```python
from build123d import *

# Parameters (mm, degrees)
SKETCH_1_R               = 13
SKETCH_1_R_2             = 12
EXTRUDE_1_DEPTH          = 6
SKETCH_2_R               = 0.75
CUT_EXTRUDE_1_DEPTH      = 14
PATTERN_CIRCULAR_1_COUNT = 16
SKETCH_3_W               = 36.79853237
SKETCH_3_H               = 11.94610836
CUT_EXTRUDE_2_DEPTH      = 14.0000001


with BuildPart() as part:
    # ｽｹｯﾁ1 → ﾎﾞｽ - 押し出し1 (new body)
    with BuildSketch(Plane.XY):
        Circle(SKETCH_1_R)
        Circle(SKETCH_1_R_2, mode=Mode.SUBTRACT)
    extrude(amount=EXTRUDE_1_DEPTH)

    # ｽｹｯﾁ2 → ｶｯﾄ - 押し出し1 (cut, through all)
    with BuildSketch(Plane(origin=(0, 0, 0), x_dir=(1, 0, 0), z_dir=(0, 1, 0))):
        with Locations((0, -3)):
            Circle(SKETCH_2_R)
    cut_extrude_1 = extrude(amount=-CUT_EXTRUDE_1_DEPTH, mode=Mode.SUBTRACT)

    # 円形ﾊﾟﾀｰﾝ1: ｶｯﾄ - 押し出し1 ×16 about axis
    pattern_circular_1_axis = Axis((0, 0, 0), (0, 0, 1))
    for i in range(1, PATTERN_CIRCULAR_1_COUNT):
        add(cut_extrude_1.rotate(pattern_circular_1_axis, i * 360 / PATTERN_CIRCULAR_1_COUNT), mode=Mode.SUBTRACT)

    # ｽｹｯﾁ3 → ｶｯﾄ - 押し出し2 (cut, through all)
    with BuildSketch(Plane(origin=(0, 0, 0), x_dir=(1, 0, 0), z_dir=(0, 1, 0))):
        with Locations((0, -2.028241391)):
            Rectangle(SKETCH_3_W, SKETCH_3_H)
    extrude(amount=-CUT_EXTRUDE_2_DEPTH, mode=Mode.SUBTRACT)


solid = part.part
```
Source: CAD feature listing. Evaluate the final solid. Frame: model axes, mm. Coordinates: 2 decimals unless noted, no trailing zeros. Loops run counter-clockwise (first coordinate to the right, second up) from the corner with the lowest first, then second, coordinate; pieces in that order, holes last. Notation, with made-up numbers: M 89,-24 L 127,-24 A13 ccw 127,-15 Z; hole C 58,-0.5 d10. An arc over 180 degrees is marked long. Put each result on its own line as item: value. Start each with the question number.
1) Ray query, L1, parallel to Z at x = 0, y = 12.6; L2, parallel to X at y = 4.75, z = 4.25; L3, parallel to X at y = 1.75, z = 1. Return the intervals inside material, ascending. Write a range as from..to.
2) Cut plane B-B on z = 3. Give the number of separate pieces and of enclosed holes in the cut face, then the cut area to 3 significant figures.
3) Contact query for flat-ended pins moving along their axis: pin 1 Ø4 at (x, y) = (9, 3.5) entering from +Z; pin 2 Ø1 at (x, z) = (7, 3.5) entering from -Y; pin 3 Ø3 at (x, y) = (-0.5, 11.5) entering from -Z; pin 4 Ø1.5 at (x, z) = (-5.5, 3) entering from -Y. Output: stop coordinate, or through.
4) Pull-direction query (Y, two-part tool) for faces 1 (the face through (0, 12, 2)), 2 (the face through (-9.33, 8.32, 2.77)), 3 (the face through (0.163, 12.481, 3.732)); classes: pulls with the +Y half, pulls with the -Y half, needs draft (parallel to the pull), parting line crosses it, or undercut.
5) Cut plane A-A on x = 0. Return the cut outline in (y, z), then the cut area to 3 significant figures.
6) Cut plane C-C on y = 1.25. Return the cut outline in (x, z), then the cut area to 3 significant figures.
7) Cut plane D-D on z = 5.5. Return the cut outline in (x, y), then the cut area to 3 significant figures.
The answers:
1. L1: z = 0..2.25, 3.75..6
1. L2: x = -12.1..-11.02, 11.02..12.1
1. L3: x = -12.88..-11.87, 11.87..12.88
2. separate pieces: 8
2. enclosed holes: 0
2. area: 27.3 mm²
3. pin 1: passes through
3. pin 2: stops at y = 9.37
3. pin 3: stops at z = 0
3. pin 4: stops at y = 10.24
4. face 1: pulls with the -Y half
4. face 2: undercut
4. face 3: needs draft
5. outline: M 12,0 L 13,0 L 13,2.25 L 12,2.25 Z; M 12,3.75 L 13,3.75 L 13,6 L 12,6 Z
5. area: 4.50 mm²
6. outline: M -12.94,0 L -11.93,0 L -11.93,6 L -12.94,6 Z; M 11.93,0 L 12.94,0 L 12.94,6 L 11.93,6 Z
6. area: 12.1 mm²
7. outline: M -13,0 L -12,0 A12 cw 12,0 L 13,0 A13 ccw Z
7. area: 39.3 mm²
